Verification items for the finished model (mm, model axes). A direction names the side the tool comes from. Coordinates: 2 decimals unless noted, no trailing zeros. Write each loop counter-clockwise with the first axis right and the second up, starting at its lowest first coordinate (ties: lowest second). Pieces come first, ordered by that corner, then holes. Notation, with made-up numbers: M 39.5,17 L 88.5,17 A17 ccw 88.5,36 Z; hole C -32,80.25 d4. An arc over 180 degrees is marked long. One line per item, written item: value.
```python
from build123d import *

# Parameters (mm, degrees)
SKETCH1_W           = 184.15
SKETCH1_H           = 184.15
SKETCH1_R           = 3.175
SKETCH1_W_2         = 34
SKETCH1_H_2         = 30
BOSS_EXTRUDE1_DEPTH = 5.9944


with BuildPart() as part:
    # Sketch1 → Boss-Extrude1 (new body)
    with BuildSketch(Plane.XY):
        with Locations((92.075, 92.075)):
            Rectangle(SKETCH1_W, SKETCH1_H)
        with Locations((9.525, 174.625)):
            Circle(SKETCH1_R, mode=Mode.SUBTRACT)
        with Locations((56.22544, 174.625)):
            Circle(SKETCH1_R, mode=Mode.SUBTRACT)
        with Locations((127.92456, 174.625)):
            Circle(SKETCH1_R, mode=Mode.SUBTRACT)
        with Locations((174.625, 174.625)):
            Circle(SKETCH1_R, mode=Mode.SUBTRACT)
        with Locations((85.725, 152.4)):
            Circle(SKETCH1_R, mode=Mode.SUBTRACT)
        with Locations((85.725, 139.7)):
            Circle(SKETCH1_R, mode=Mode.SUBTRACT)
        with Locations((9.525, 9.525)):
            Circle(SKETCH1_R, mode=Mode.SUBTRACT)
        with Locations((85.725, 44.45)):
            Circle(SKETCH1_R, mode=Mode.SUBTRACT)
        with Locations((56.22544, 9.525)):
            Circle(SKETCH1_R, mode=Mode.SUBTRACT)
        with Locations((85.725, 31.75)):
            Circle(SKETCH1_R, mode=Mode.SUBTRACT)
        with Locations((127.92456, 9.525)):
            Circle(SKETCH1_R, mode=Mode.SUBTRACT)
        with Locations((174.61738, 9.525)):
            Circle(SKETCH1_R, mode=Mode.SUBTRACT)
        with Locations((32.87522, 149.76218)):
            Rectangle(SKETCH1_W_2, SKETCH1_H_2, mode=Mode.SUBTRACT)
        with Locations((32.87522, 34.38782)):
            Rectangle(SKETCH1_W_2, SKETCH1_H_2, mode=Mode.SUBTRACT)
        with Locations((151.27478, 149.76218)):
            Rectangle(SKETCH1_W_2, SKETCH1_H_2, mode=Mode.SUBTRACT)
        with Locations((151.27478, 34.38782)):
            Rectangle(SKETCH1_W_2, SKETCH1_H_2, mode=Mode.SUBTRACT)
    extrude(amount=BOSS_EXTRUDE1_DEPTH)


solid = part.part
```
Item 1: Cross-section at A-A, the plane x = 161.5. Enter the section's corners in (y, z).
The answers:
outline: M 0,0 L 19.39,0 L 19.39,5.99 L 0,5.99 Z; M 49.39,0 L 134.76,0 L 134.76,5.99 L 49.39,5.99 Z; M 164.76,0 L 184.15,0 L 184.15,5.99 L 164.76,5.99 Z
Item 2: Access from +Z, -Z, +X, -X, +Y, -Y to the whole of each face (thin tool, end or side, straight path). Record for faces 1 (the face through (184.15, 91, 3)), 2 (the face through (33, 164.762, 3)).
The answers:
face 1: +Z, -Z, +X, +Y, -Y
face 2: +Z, -Z
Item 3: Go/stop test with flat-tipped pins: P1, Ø7.5, axis at x = 174.62, y = 9.52, coming from the -Z side; P2, Ø5.5, axis at x = 56.23, y = 174.62, coming from the +Z side. Record where each tip stops, or that it passes through.
The answers:
P1: stops at z = 0
P2: passes through
Item 4: Cross-section at C-C, the plane z = 1.4. Give the number of separate pieces and of enclosed holes in the cut face, and give its area (3 significant figures).
The answers:
separate pieces: 1
enclosed holes: 16
area: 29,500 mm²
Item 5: Scan lines: line 1 (X direction, y = 9.5, z = 0.3); line 2 (X direction, y = 152.4, z = 3); line 3 (Y direction, x = 26.5, z = 1.55). Record each from-to range of solid material in increasing order.
The answers:
line 1: x = 0 to 6.35, 12.7 to 53.05, 59.4 to 124.75, 131.1 to 171.44, 177.79 to 184.15
line 2: x = 0 to 15.88, 49.88 to 82.55, 88.9 to 134.27, 168.27 to 184.15
line 3: y = 0 to 19.39, 49.39 to 134.76, 164.76 to 184.15
Item 6: Cross-section at B-B, the plane y = 44.45. Enter the section's corners in (x, z).
The answers:
outline: M 0,0 L 15.88,0 L 15.88,5.99 L 0,5.99 Z; M 49.88,0 L 82.55,0 L 82.55,5.99 L 49.88,5.99 Z; M 88.9,0 L 134.27,0 L 134.27,5.99 L 88.9,5.99 Z; M 168.27,0 L 184.15,0 L 184.15,5.99 L 168.27,5.99 Z
